Geometry check sheet. Reference: the model listing, model coordinates, mm. A direction names the side the tool comes from. Coordinates: 2 decimals unless noted, no trailing zeros. Write each loop counter-clockwise with the first axis right and the second up, starting at its lowest first coordinate (ties: lowest second). Pieces come first, ordered by that corner, then holes. Notation, with made-up numbers: (73.25, 86.25) -> (100.25, 86.25) arc R21 cw to (100.25, 105.25) -> close; hole circle Ø7 at (1, 71.5). An arc over 180 degrees is marked (long way). Answer in a Markdown table with one row per item. Add a question column.
1. Cross-section at D-D on y = -7.5. Record the cut outline in (x, z), and give its area (3 significant figures).
2. Mould release check, pull along Z, two halves, no side actions. Record for faces 1 (the flat face through (0, 0, 38.1)), 2 (the flat face through (-4.8, -15.5, 0)), 3 (the cylindrical face through (-0.089, -2.753, 10.448)), 4 (the flat face through (-6.35, 7, 11)): pulls with the +Z half, pulls with the -Z half, needs draft (parallel to the pull), parting line crosses it, or undercut.
3. Cross-section at C-C on x = 5.5. Record the cut outline in (y, z) (3 decimals).
4. Cross-section at B-B on z = 12.5. Record the cut outline in (x, y) (3 decimals).
5. Depth check by flat-ended pin: P1, Ø1, axis at y = 10, z = 30, coming from the -X side; P2, Ø6, axis at x = -9.5, y = 1, coming from the +Z side; P3, Ø1, axis at x = 3.5, y = -10.5, coming from the -Z side. Enter the tip coordinate at first touch or a pass-through.
6. Scan lines: L1, parallel to Y at x = 0, z = -9 (3 decimals); L2, parallel to Z at x = 2.5, y = 0; L3, parallel to X at y = 8.5, z = 8. Record each from-to range of solid material in increasing order. Write a range as from..to.
7. Cross-section at A-A on y = 0. Record the cut outline in (x, z) (3 decimals).
8. Set-up check for faces 5 (the flat face through (4.6, -15.4, 0)), 6 (the flat face through (10, 0, 0)), 7 (the cylindrical face through (-2.75, 12.4, -9.57)): record each of +Z, -Z, +X, -X, +Y, -Y from which the full face is reachable in a straight line by a thin tool's end or side.
```python
from build123d import *

# Parameters (mm, degrees)
F0_R     = 12.7
F2_DEPTH = 6.35
F3_DEPTH = 6.35
F1_R     = 15.875
F1_R_2   = 12.7
F4_DEPTH = 12.7
F5_R     = 12.7
F6_DEPTH = 6.35


with BuildPart() as f2:
    # F0 (on Right) → F2 (new body)
    with BuildSketch(Plane.YZ):
        with BuildLine():
            Line((-15.875, 0), (15.875, 0))
            Line((15.875, 0), (15.875, 31.75))
            ThreePointArc((15.875, 31.75), (14.0151280605, 36.2401280605), (9.525, 38.1))
            Line((9.525, 38.1), (-9.525, 38.1))
            ThreePointArc((-9.525, 38.1), (-14.0151280605, 36.2401280605), (-15.875, 31.75))
            Line((-15.875, 31.75), (-15.875, 0))
        make_face()
        with Locations((0, 22.8458158672)):
            Circle(F0_R, mode=Mode.SUBTRACT)
    extrude(amount=F2_DEPTH)

    # F3 (add): a face of the model
    f3_faces = [f2.faces().sort_by_distance(p)[0] for p in [
        (0, 0, 0.4959508544),
    ]]
    extrude(f3_faces, amount=F3_DEPTH)

    # F1 (on Top) → F4 (join)
    with BuildSketch(Plane.XY):
        Circle(F1_R)
        Circle(F1_R_2, mode=Mode.SUBTRACT)
        Circle(F1_R_2)
    extrude(amount=-F4_DEPTH)

    # F5 (on face) → F6 (cut)
    with BuildSketch(Plane(origin=(0, 0, -12.7), x_dir=(1, 0, 0), z_dir=(0, 0, -1))):
        Circle(F5_R)
    extrude(amount=-F6_DEPTH, mode=Mode.SUBTRACT)


solid = f2.part
```
Results found:
| question | item | result |
|---|---|---|
| 1 | outline | (-13.99, -12.7) -> (-10.25, -12.7) -> (-10.25, -6.35) -> (10.25, -6.35) -> (10.25, -12.7) -> (13.99, -12.7) -> (13.99, 0) -> (6.35, 0) -> (6.35, 12.6) -> (-6.35, 12.6) -> (-6.35, 0) -> (-13.99, 0) -> close; (-6.35, 33.09) -> (6.35, 33.09) -> (6.35, 38.1) -> (-6.35, 38.1) -> close |
| 1 | area | 449 mm^2 |
| 2 | face 1 | pulls with the +Z half |
| 2 | face 2 | pulls with the -Z half |
| 2 | face 3 | undercut |
| 2 | face 4 | needs draft |
| 3 | outline | (-15.875, 0) -> (-14.892, 0) -> (-14.892, -12.7) -> (-11.447, -12.7) -> (-11.447, -6.35) -> (11.447, -6.35) -> (11.447, -12.7) -> (14.892, -12.7) -> (14.892, 0) -> (15.875, 0) -> (15.875, 31.75) arc R6.35 ccw to (9.525, 38.1) -> (-9.525, 38.1) arc R6.35 ccw to (-15.875, 31.75) -> close; hole circle Ø25.4 at (0, 22.846) |
| 4 | outline | (-6.35, -15.875) -> (6.35, -15.875) -> (6.35, -7.366) -> (-6.35, -7.366) -> close; (-6.35, 7.366) -> (6.35, 7.366) -> (6.35, 15.875) -> (-6.35, 15.875) -> close |
| 5 | P1 | stops at x = -6.35 |
| 5 | P2 | stops at z = 0 |
| 5 | P3 | stops at z = -6.35 |
| 6 | L1 | y = -15.875..-12.7, 12.7..15.875 |
| 6 | L2 | z = -6.35..10.15, 35.55..38.1 |
| 6 | L3 | x = -6.35..6.35 |
| 7 | outline | (-15.875, -12.7) -> (-12.7, -12.7) -> (-12.7, -6.35) -> (12.7, -6.35) -> (12.7, -12.7) -> (15.875, -12.7) -> (15.875, 0) -> (6.35, 0) -> (6.35, 10.146) -> (-6.35, 10.146) -> (-6.35, 0) -> (-15.875, 0) -> close; (-6.35, 35.546) -> (6.35, 35.546) -> (6.35, 38.1) -> (-6.35, 38.1) -> close |
| 8 | face 5 | -Z, +X, -Y |
| 8 | face 6 | +Z, +X, +Y, -Y |
| 8 | face 7 | -Z |
